Here's how the part is built. I have some questions about the finished solid (model axes, mm). A direction names the side the tool comes from. Coordinates: 2 decimals unless noted, no trailing zeros. Write each loop counter-clockwise with the first axis right and the second up, starting at its lowest first coordinate (ties: lowest second). Pieces come first, ordered by that corner, then holes.
Item 1: I'm going to push flat-ended pins straight in: pin 1 Ø0.8 at (y, z) = (27, 1) entering from -X; pin 2 Ø0.8 at (x, z) = (13.5, 1) entering from -Y. Where does each tip first touch, or does it pass through?
Item 2: If we section it at A-A (z = 1.3): Count the separate pieces of the cut face and the enclosed holes in it, then the cut area to 3 significant figures.
Item 3: If we section it at B-B (y = 22): Please give me the cut outline in (x, z), then the cut area to 3 significant figures.
Item 4: If I drill on line 1 (Y direction, x = 62.5, z = 0.6); line 2 (Y direction, x = 19.5, z = 0.6); line 3 (X direction, y = 15.5, z = 0.8), over which ranges is the centre line in solid material (lowest first)?
Item 5: For faces 5 (the face through (12, 20.675, 1)), 6 (the face through (36, 15, 1.6)), which set-ups out of +Z, -Z, +X, -X, +Y, -Y let a thin tool reach every point of the face, with its end or its side?
Item 6: We'd pull the mould along X, two halves only. Please class faces 1 (the face through (61.22, 26.72, 0.81)), 2 (the face through (12, 8.675, 1)), 3 (the face through (16.317, -1, 1)), 4 (the face through (57.672, 13.317, 0.811)): +X half, -X half, draft (parallel to the pull), parting line (faces both ways), or undercut.
from build123d import *

# Parameters (mm, degrees)
F0_W     = 9
F0_H     = 12
F0_W_2   = 50
F0_H_2   = 19
F1_DEPTH = 1.6
F4_R     = 0.35
F5_R     = 0.35
F2_R     = 0.35
F6_DEPTH = 4
F7_R     = 1.1
F8_DEPTH = 25


# Not quite as in the source:
# - a feature names something its author has since deleted; it is built from what else it names


with BuildPart() as f1:
    # F0 (on Top) → F1 (new body)
    with BuildSketch(Plane.XY):
        with Locations((11.8172904253, 14.6750973295)):
            Rectangle(F0_W, F0_H)
        with Locations((41.3172904253, 14.6750973295)):
            Rectangle(F0_W_2, F0_H)
        with Locations((41.3172904253, -0.8249026705)):
            Rectangle(F0_W_2, F0_H_2)
        with Locations((41.3172904253, 30.1750973295)):
            Rectangle(F0_W_2, F0_H_2)
    extrude(amount=F1_DEPTH)

    # F4 (on face) + F5 (on face) + F3 (on face) + F2 (on face) → F6 (cut)
    with BuildSketch(Plane.XY.offset(1.6)):
        with Locations((51.6172904253, 6.6970097786)):
            Circle(F4_R)
        with Locations((56.6172904253, 6.6970097786)):
            Circle(F4_R)
        with Locations((54.1172904253, 6.6970097786)):
            Circle(F4_R)
    with BuildSketch(Plane.XY.offset(1.6)):
        with Locations((8.5672904253, 14.6970097786)):
            Circle(F5_R)
        with Locations((12.0672904253, 14.6970097786)):
            Circle(F5_R)
    with BuildSketch(Plane.XY.offset(1.6)):
        with BuildLine():
            Line((54.8172904253, 15.4470097786), (53.8172904253, 15.4470097786))
            ThreePointArc((53.8172904253, 15.4470097786), (53.640513733, 15.5202330803), (53.5672904253, 15.6970097701))
            ThreePointArc((53.5672904253, 15.6970097701), (54.3172904296, 14.9470097786), (55.0672904253, 15.6970097786))
            ThreePointArc((55.0672904253, 15.6970097786), (54.9940671206, 15.5202330833), (54.8172904253, 15.4470097786))
        make_face()
        with BuildLine():
            ThreePointArc((53.5672904253, 15.6970097701), (53.640513733, 15.5202330803), (53.8172904253, 15.4470097786))
            Line((53.8172904253, 15.4470097786), (54.8172904253, 15.4470097786))
            ThreePointArc((54.8172904253, 15.4470097786), (54.9940671206, 15.5202330833), (55.0672904253, 15.6970097786))
            ThreePointArc((55.0672904253, 15.6970097786), (54.9940671206, 15.8737864739), (54.8172904253, 15.9470097786))
            Line((54.8172904253, 15.9470097786), (53.8172904253, 15.9470097786))
            ThreePointArc((53.8172904253, 15.9470097786), (53.640513727, 15.8737864709), (53.5672904253, 15.6970097701))
        make_face()
        with BuildLine():
            ThreePointArc((55.0672904253, 15.6970097786), (54.317290421, 16.4470097786), (53.5672904253, 15.6970097701))
            ThreePointArc((53.5672904253, 15.6970097701), (53.640513727, 15.8737864709), (53.8172904253, 15.9470097786))
            Line((53.8172904253, 15.9470097786), (54.8172904253, 15.9470097786))
            ThreePointArc((54.8172904253, 15.9470097786), (54.9940671206, 15.8737864739), (55.0672904253, 15.6970097786))
        make_face()
        with BuildLine():
            Line((51.1672904253, 13.7970097786), (51.8672904253, 13.7970097786))
            ThreePointArc((51.8672904253, 13.7970097786), (52.0440671206, 13.7237864739), (52.1172904253, 13.5470097786))
            ThreePointArc((52.1172904253, 13.5470097786), (51.5172904253, 14.1470097786), (50.9172904253, 13.5470097786))
            ThreePointArc((50.9172904253, 13.5470097786), (50.99051373, 13.7237864739), (51.1672904253, 13.7970097786))
        make_face()
        with BuildLine():
            ThreePointArc((52.1172904253, 13.5470097786), (52.0440671206, 13.7237864739), (51.8672904253, 13.7970097786))
            Line((51.8672904253, 13.7970097786), (51.1672904253, 13.7970097786))
            ThreePointArc((51.1672904253, 13.7970097786), (50.99051373, 13.7237864739), (50.9172904253, 13.5470097786))
            ThreePointArc((50.9172904253, 13.5470097786), (50.99051373, 13.3702330833), (51.1672904253, 13.2970097786))
            Line((51.1672904253, 13.2970097786), (51.8672904253, 13.2970097786))
            ThreePointArc((51.8672904253, 13.2970097786), (52.0440671206, 13.3702330833), (52.1172904253, 13.5470097786))
        make_face()
        with BuildLine():
            ThreePointArc((50.9172904253, 13.5470097786), (51.5172904253, 12.9470097786), (52.1172904253, 13.5470097786))
            ThreePointArc((52.1172904253, 13.5470097786), (52.0440671206, 13.3702330833), (51.8672904253, 13.2970097786))
            Line((51.8672904253, 13.2970097786), (51.1672904253, 13.2970097786))
            ThreePointArc((51.1672904253, 13.2970097786), (50.99051373, 13.3702330833), (50.9172904253, 13.5470097786))
        make_face()
        with BuildLine():
            Line((56.7672904253, 13.2970097786), (57.4672904253, 13.2970097786))
            ThreePointArc((57.4672904253, 13.2970097786), (57.6440671206, 13.3702330833), (57.7172904253, 13.5470097786))
            ThreePointArc((57.7172904253, 13.5470097786), (57.6440671206, 13.7237864739), (57.4672904253, 13.7970097786))
            Line((57.4672904253, 13.7970097786), (56.7672904253, 13.7970097786))
            ThreePointArc((56.7672904253, 13.7970097786), (56.59051373, 13.7237864739), (56.5172904253, 13.5470097786))
            ThreePointArc((56.5172904253, 13.5470097786), (56.59051373, 13.3702330833), (56.7672904253, 13.2970097786))
        make_face()
        with BuildLine():
            ThreePointArc((57.7172904253, 13.5470097786), (57.6440671206, 13.3702330833), (57.4672904253, 13.2970097786))
            Line((57.4672904253, 13.2970097786), (56.7672904253, 13.2970097786))
            ThreePointArc((56.7672904253, 13.2970097786), (56.59051373, 13.3702330833), (56.5172904253, 13.5470097786))
            ThreePointArc((56.5172904253, 13.5470097786), (57.1172904253, 12.9470097786), (57.7172904253, 13.5470097786))
        make_face()
        with BuildLine():
            ThreePointArc((57.4672904253, 13.7970097786), (57.6440671206, 13.7237864739), (57.7172904253, 13.5470097786))
            ThreePointArc((57.7172904253, 13.5470097786), (57.1172904253, 14.1470097786), (56.5172904253, 13.5470097786))
            ThreePointArc((56.5172904253, 13.5470097786), (56.59051373, 13.7237864739), (56.7672904253, 13.7970097786))
            Line((56.7672904253, 13.7970097786), (57.4672904253, 13.7970097786))
        make_face()
    with BuildSketch(Plane.XY.offset(1.6)):
        with Locations((27.3172904253, 15.6970097786)):
            Circle(F2_R)
        with Locations((29.3172904253, 15.6970097786)):
            Circle(F2_R)
        with Locations((31.3172904253, 15.6970097786)):
            Circle(F2_R)
    extrude(amount=-F6_DEPTH, mode=Mode.SUBTRACT)

    # F7 (on face) → F8 (cut)
    with BuildSketch(Plane.XY.offset(1.6)):
        with Locations((62.3172904253, 26.6750973295)):
            Circle(F7_R)
        with Locations((20.3172904253, 26.6750973295)):
            Circle(F7_R)
        with Locations((62.3172904253, 2.6750973295)):
            Circle(F7_R)
        with Locations((20.3172904253, 2.6750973295)):
            Circle(F7_R)
        with Locations((41.3172904253, 2.6750973295)):
            Circle(F7_R)
        with Locations((41.3172904253, 26.6750973295)):
            Circle(F7_R)
    extrude(amount=-F8_DEPTH, mode=Mode.SUBTRACT)


solid = f1.part
Answer list:
1. pin 1: stops at x = 16.32
1. pin 2: stops at y = 8.68
2. separate pieces: 1
2. enclosed holes: 17
2. area: 2,580 mm2
3. outline: (16.32, 0) - (66.32, 0) - (66.32, 1.6) - (16.32, 1.6) - close
3. area: 80.0 mm2
4. line 1: y = -10.32 to 1.59, 3.76 to 25.59, 27.76 to 39.68
4. line 2: y = -10.32 to 1.94, 3.41 to 25.94, 27.41 to 39.68
4. line 3: x = 7.32 to 27.03, 27.61 to 29.03, 29.61 to 31.03, 31.61 to 53.59, 55.04 to 66.32
5. face 5: +Z, -Z, -X, +Y
5. face 6: +Z, +X, -X, +Y, -Y
6. face 1: undercut
6. face 2: draft
6. face 3: -X half
6. face 4: undercut
